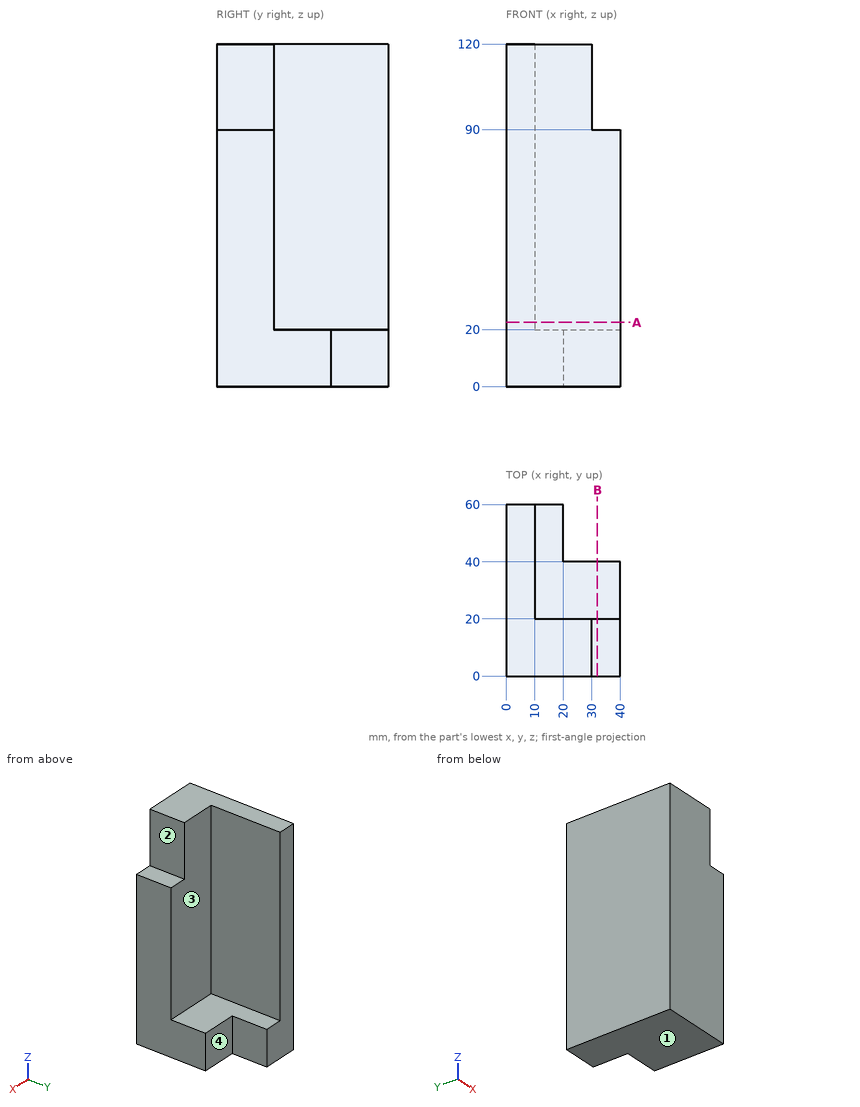
Study the drawing (mm; zero at the part's minimum x, y, z) and answer. A direction names the side the tool comes from. Round coordinates to 2 decimals unless told otherwise and drop trailing zeros. Write each loop counter-clockwise with the first axis right and the second up, starting at its lowest first coordinate (ties: lowest second). Pieces come first, ordered by that corner, then holes. Notation, with made-up numbers: (28, 1.5) -> (33, 1.5) arc R15 ccw to (33, 13.5) -> close; hole circle Ø1 at (56, 67.25). An arc over 180 degrees is marked (long way). Use CSV: the item, a comma, the result in double quotes. Start each with the question number.
(1) Each of these flat-tipped pins is pushed along its axis until it touches: pin 1 (3 mm diameter, centred on y = 35, z = 94, fed in from -X); pin 2 (3 mm diameter, centred on x = 34.5, y = 14.5, fed in from +Z); pin 3 (6 mm diameter, centred on y = 14.5, z = 100.5, fed in from +X); pin 4 (10 mm diameter, centred on y = 52, z = 7.5, fed in from +X). Where does it stop, or does it pass through?
(2) Section A-A on z = 22.5 is taken. Give the vertices of the cut face in (x, y).
(3) Section B-B on x = 32 is taken. Give the vertices of the cut face in (y, z).
(4) Which of the six approach directions +Z, -Z, +X, -X, +Y, -Y give full straight-line access (tool end or side, diameter ignored) to the marked faces 1, 2, 3 and 4?
(5) Consider L1, parallel to X at y = 55, z = 94; L2, parallel to X at y = 5, z = 98; L3, parallel to Y at x = 16, z = 45.5. Determine where each line is inside the solid, lowest interval first. Write a range as from..to.
A:
1,pin 1,"stops at x = 0"
1,pin 2,"stops at z = 90"
1,pin 3,"stops at x = 30"
1,pin 4,"stops at x = 20"
2,outline,"(0, 0) -> (40, 0) -> (40, 20) -> (10, 20) -> (10, 60) -> (0, 60) -> close"
3,outline,"(0, 0) -> (40, 0) -> (40, 20) -> (20, 20) -> (20, 90) -> (0, 90) -> close"
4,face 1,"-Z, +X, -X, +Y, -Y"
4,face 2,"+Z, +X, +Y, -Y"
4,face 3,"+Z, +X, +Y"
4,face 4,"+Z, -Z, +X, +Y"
5,L1,"x = 0..10"
5,L2,"x = 0..30"
5,L3,"y = 0..20"
